Autodesk Inventor part; units mm, degrees
ref_plane "YZ Plane" through (0, 0, 0) normal (1, 0, 0) x (0, 1, 0)
ref_plane "XZ Plane" through (0, 0, 0) normal (0, 1, 0) x (-1, 0, 0)
ref_plane "XY Plane" through (0, 0, 0) normal (0, 0, 1) x (1, 0, 0)
sketch "Sketch1" plane through (0, 0, 0) normal (0, 1, 0) x (-1, 0, 0)
  circle A0 centre (8, 0) radius 3
  line L0 (8, 0) -> (-8, 0)
  circle A1 centre (-8, 0) radius 3
  arc A2 (6.1538, -2.3647) -> (-6.1538, -2.3647) centre (0, -10.247) ccw
  line L1 (0, -0.247) -> (0, 5.753)
  arc A3 (9.8462, 2.3647) -> (-9.8462, 2.3647) centre (0, -10.247) ccw
  circle A4 centre (8, 0) radius 1.5
  circle A5 centre (-8, 0) radius 1.5
  point P0 (0, 0)
  dimension "d13" = 16
  dimension "d14" = 6
  dimension "d16" = 6
  dimension "d17" = 3
  dimension "d18" = 3
extrude "Extrusion1" add sketch "Sketch1" along normal blind 2
sketch "Sketch2" plane through (0, 0, 0) normal (0, -1, 0) x (1, 0, 0)
  circle A0 centre (8, 0) radius 1.5
  circle A1 centre (-8, 0) radius 1.5
  arc A2 (6.1538, -2.3647) -> (9.8462, 2.3647) centre (8, 0) ccw
  arc A3 (-9.8462, 2.3647) -> (-6.1538, -2.3647) centre (-8, 0) ccw
  circle A4 centre (-8, 0) radius 0.05
  circle A5 centre (8, 0) radius 0.05
  point P0 (0, 0)
  dimension "d21" = 0.1
  dimension "d22" = 0.1
extrude "Extrusion2" add sketch "Sketch2" against normal blind 2
properties part number "tahlo-neco_sablona"
Work out the finished part from the listing and answer in its coordinate system (mm). Coordinates: 2 decimals unless noted, no trailing zeros. Loops run counter-clockwise (first coordinate to the right, second up) from the corner with the lowest first, then second, coordinate; pieces in that order, holes last. Notation, with made-up numbers: M 2.25,-34 L 8.25,-34 A15 ccw 8.25,-5 Z; hole C -20.5,-14 d3. An arc over 180 degrees is marked long. Answer in a Markdown table with one row per item. Add a question column.
1. Consider L1, parallel to X at y = 1.1, z = -1; L2, parallel to X at y = 1.3, z = 3.5; L3, parallel to X at y = 0.75, z = -2.5. Determine where each line is inside the solid, lowest interval first.
2. The mould has two halves that part along X. Classify faces 1 (the cylindrical face through (0.148, 0.986, 5.752)), 2 (the cylindrical face through (0.093, 0.986, -0.247)), 3 (the flat face through (0, 2, 1)): pulls with the +X half, pulls with the -X half, needs draft (parallel to the pull), parting line crosses it, or undercut.
3. Find section A-A, the plane z = -2. Write down the section's boundary in (x, y), then the cut area to 3 significant figures.
4. Find section C-C, the plane x = -7.25. Write down the section's boundary in (y, z).
5. Find section D-D, the plane z = 1.5. Write down the section's boundary in (x, y).
6. Flat-ended cylindrical pins translate along their axes: P1, Ø3, axis at x = 3, z = 2.5, coming from the -Y side; P2, Ø1, axis at y = 0, z = -1.5, coming from the -X side. Find the tip coordinate at first contact, or state that the pin passes through.
Reported:
| question | item | result |
|---|---|---|
| 1 | L1 | x = -10.83 to -3.81, 3.81 to 10.83 |
| 1 | L2 | x = -8.19 to 8.19 |
| 1 | L3 | x = -9.66 to -6.34, 6.34 to 9.66 |
| 2 | face 1 | parting line crosses it |
| 2 | face 2 | undercut |
| 2 | face 3 | needs draft |
| 3 | outline | M -10.24,0 L -5.66,0 L -5.66,2 L -10.24,2 Z; M 5.66,0 L 10.24,0 L 10.24,2 L 5.66,2 Z |
| 3 | area | 18.3 mm^2 |
| 4 | outline | M 0,-2.9 L 2,-2.9 L 2,4.02 L 0,4.02 Z |
| 5 | outline | M -10.6,0 L 10.6,0 L 10.6,2 L -10.6,2 Z |
| 6 | P1 | stops at y = 0 |
| 6 | P2 | stops at x = -10.83 |
